from build123d import *

# Parameters (mm, degrees)
F1_DEPTH = 19.05
F2_DEPTH = 19.05
F3_W     = 12.7
F3_H     = 19.05
F4_DEPTH = 25.4
F6_DEPTH = 6.35
F8_DEPTH = 6.35


with BuildPart() as f1:
    # F0 (on Right) → F1 (new body, symmetric)
    with BuildSketch(Plane.YZ):
        Polygon((-12.7, 0), (0, 0), (0, 25.4), (-12.7, 12.7), (-12.7, 6.35), align=None)
        Polygon((-25.4, 0), (-12.7, 0), (-12.7, 6.35), (-19.05, 6.35), align=None)
        Polygon((-12.7, 6.35), (-12.7, 12.7), (-19.05, 6.35), align=None)
        Polygon((-25.4, 6.35), (-25.4, 0), (-19.05, 6.35), align=None)
    extrude(amount=F1_DEPTH, both=True)

    # F0 (on Right) → F2 (cut)
    with BuildSketch(Plane.YZ):
        Polygon((-12.7, 6.35), (-12.7, 12.7), (-19.05, 6.35), align=None)
        Polygon((-25.4, 6.35), (-25.4, 0), (-19.05, 6.35), align=None)
        Polygon((-25.4, 0), (-12.7, 0), (-12.7, 6.35), (-19.05, 6.35), align=None)
    extrude(amount=F2_DEPTH, mode=Mode.SUBTRACT)

    # F3 (on face) → F4 (cut)
    with BuildSketch(Plane(origin=(0, 0, 0), x_dir=(-1, 0, 0), z_dir=(0, 1, 0))):
        with Locations((6.35, 15.875)):
            Rectangle(F3_W, F3_H)
    extrude(amount=-F4_DEPTH, mode=Mode.SUBTRACT)

    # F5 (on face) → F6 (cut)
    with BuildSketch(Plane(origin=(-19.05, 0, 0), x_dir=(0, -1, 0), z_dir=(-1, 0, 0))):
        Polygon((25.4, 6.35), (19.05, 6.35), (25.4, 0), align=None)
    extrude(amount=-F6_DEPTH, mode=Mode.SUBTRACT)

    # F7 (on face) → F8 (cut, through all)
    with BuildSketch(Plane.XY.offset(6.35)):
        with BuildLine():
            ThreePointArc((-3.175, -6.35), (-6.35, -3.175), (-9.525, -6.35))
            Line((-9.525, -6.35), (-9.525, -19.05))
            ThreePointArc((-9.525, -19.05), (-6.35, -22.225), (-3.175, -19.05))
            Line((-3.175, -19.05), (-3.175, -6.35))
        make_face()
    extrude(amount=-F8_DEPTH, mode=Mode.SUBTRACT)


solid = f1.part
Verification items for the finished model (mm, model axes). A direction names the side the tool comes from. Coordinates: 2 decimals unless noted, no trailing zeros. Write each loop counter-clockwise with the first axis right and the second up, starting at its lowest first coordinate (ties: lowest second). Pieces come first, ordered by that corner, then holes. Notation, with made-up numbers: (-28.5, -20) -> (9.5, -20) arc R20 ccw to (9.5, 18) -> close; hole circle Ø8 at (26, 6.5). An arc over 180 degrees is marked (long way). One line per item, written item: value. Start each with the question number.
Q1. Access from +Z, -Z, +X, -X, +Y, -Y to the whole of each face (thin tool, end or side, straight path). Record for faces 1 (the flat face through (-15.8, -12.5, 12.9)), 2 (the flat face through (9, -12.7, 6)), 3 (the cylindrical face through (-6.28, -3.176, 3.219)).
Q2. Cross-section at C-C on z = 4.5. Enter the section's corners in (x, y) (3 decimals).
Q3. Go/stop test with flat-tipped pins: P1, Ø10, axis at x = 3, y = -16, coming from the +Z side; P2, Ø1.5, axis at x = -11, y = -12.5, coming from the +Z side; P3, Ø1, axis at x = 14.5, y = -14, coming from the +Z side; P4, Ø3, axis at y = -20.5, z = 2, coming from the +X side. Record where each tip stops, or that it passes through.
Q4. Thickness scan on L1, parallel to X at y = -4, z = 18.75; L2, parallel to X at y = -10, z = 6 (3 decimals); L3, parallel to Z at x = -2, y = -21.25. Record the ranges inside material, lowest first. Write a range as from..to.
Q5. Cross-section at B-B on z = 23. Enter the section's corners in (x, y).
Q6. Cross-section at D-D on x = -6.35. Enter the section's corners in (y, z) (3 decimals).
Q7. Cross-section at A-A on y = -10.75. Enter the section's corners in (x, z) (3 decimals), and give its area (3 significant figures).
Q8. Mould release check, pull along X, two halves, no side actions. Record for faces 4 (the flat face through (-6, -25.4, 3)), 5 (the flat face through (-3.175, -13, 3)), 6 (the flat face through (-12.7, -24, 5)), 7 (the flat face through (-12.7, -7, 14)): pulls with the +X half, pulls with the -X half, needs draft (parallel to the pull), parting line crosses it, or undercut.
Checked values:
1. face 1: +Z, -X, -Y
1. face 2: +Z, -Z, +X, -Y
1. face 3: +Z, -Z
2. outline: (-19.05, -20.9) -> (-12.7, -20.9) -> (-12.7, -25.4) -> (0, -25.4) -> (0, -12.7) -> (19.05, -12.7) -> (19.05, 0) -> (-19.05, 0) -> close; hole (-9.525, -19.05) arc R3.175 ccw to (-3.175, -19.05) -> (-3.175, -6.35) arc R3.175 ccw to (-9.525, -6.35) -> close
3. P1: stops at z = 14.4
3. P2: stops at z = 6.35
3. P3: passes through
3. P4: stops at x = 0
4. L1: x = -19.05..-12.7, 0..19.05
4. L2: x = -19.05..-9.525, -3.175..19.05
4. L3: z = 0..6.35
5. outline: (-19.05, -2.4) -> (-12.7, -2.4) -> (-12.7, 0) -> (-19.05, 0) -> close; (0, -2.4) -> (19.05, -2.4) -> (19.05, 0) -> (0, 0) -> close
6. outline: (-25.4, 0) -> (-22.225, 0) -> (-22.225, 6.35) -> (-25.4, 6.35) -> close; (-3.175, 0) -> (0, 0) -> (0, 6.35) -> (-3.175, 6.35) -> close
7. outline: (-19.05, 0) -> (-9.525, 0) -> (-9.525, 6.35) -> (-12.7, 6.35) -> (-12.7, 14.65) -> (-19.05, 14.65) -> close; (-3.175, 0) -> (19.05, 0) -> (19.05, 14.65) -> (0, 14.65) -> (0, 6.35) -> (-3.175, 6.35) -> close
7. area: 412 mm²
8. face 4: needs draft
8. face 5: undercut
8. face 6: pulls with the -X half
8. face 7: undercut
